from build123d import *

# Parameters (mm, degrees)
CLONE2D_W                = 34.6
CLONE2D_H                = 34.6
PAD004_DEPTH             = 1.2
SKETCH019_W              = 33
SKETCH019_H              = 33
PAD005_DEPTH             = 1.6
PAD006_DEPTH             = 3.3
SKETCH021_W              = 8
SKETCH021_H              = 22.4
SKETCH021_W_2            = 22.4
SKETCH021_H_2            = 5
SKETCH021_W_3            = 10
SKETCH021_H_3            = 9
POCKET014_DEPTH          = 1.2
SKETCH022_R              = 2.5
POCKET015_DEPTH          = 0.5
SKETCH023_R              = 1.25
POCKET016_DEPTH          = 6.101
SKETCH024_W              = 10.5
SKETCH024_H              = 4.5
SKETCH024_W_2            = 4.5
SKETCH024_H_2            = 8
SKETCH024_H_3            = 7
POCKET017_DEPTH          = 2.801
CLONE002_PLACEMENT_ANGLE = 180


with BuildPart() as part:
    # Clone2D → Pad004 (new body)
    with BuildSketch(Plane.XY):
        Rectangle(CLONE2D_W, CLONE2D_H)
    extrude(amount=PAD004_DEPTH)

    # Sketch019 → Pad005 (new body)
    with BuildSketch(Plane.XY.offset(1.2)):
        Rectangle(SKETCH019_W, SKETCH019_H)
    extrude(amount=PAD005_DEPTH)

    # Sketch020 → Pad006 (new body)
    with BuildSketch(Plane.XY.offset(2.8)):
        with BuildLine():
            ThreePointArc((-14, 11.5), (-12.232233, 12.232233), (-11.5, 14))
            Line((-11.5, 16.5), (-11.5, 14))
            Line((-11.5, 16.5), (-16.5, 16.5))
            Line((-16.5, 16.5), (-16.5, 11.5))
            Line((-16.5, 11.5), (-14, 11.5))
        make_face()
        with BuildLine():
            ThreePointArc((11.5, 14), (12.232233, 12.232233), (14, 11.5))
            Line((14, 11.5), (16.5, 11.5))
            Line((16.5, 11.5), (16.5, 16.5))
            Line((16.5, 16.5), (11.5, 16.5))
            Line((11.5, 16.5), (11.5, 14))
        make_face()
        with BuildLine():
            ThreePointArc((-11.5, -14), (-12.232233, -12.232233), (-14, -11.5))
            Line((-16.5, -11.5), (-14, -11.5))
            Line((-16.5, -16.5), (-16.5, -11.5))
            Line((-11.5, -16.5), (-16.5, -16.5))
            Line((-11.5, -14), (-11.5, -16.5))
        make_face()
        with BuildLine():
            ThreePointArc((14, -11.5), (12.232233, -12.232233), (11.5, -14))
            Line((11.5, -14), (11.5, -16.5))
            Line((11.5, -16.5), (16.5, -16.5))
            Line((16.5, -16.5), (16.5, -11.5))
            Line((16.5, -11.5), (14, -11.5))
        make_face()
    extrude(amount=PAD006_DEPTH)

    # Sketch021 → Pocket014 (cut)
    with BuildSketch(Plane.XY.offset(2.8)):
        with Locations((12.5, 0)):
            Rectangle(SKETCH021_W, SKETCH021_H)
        with Locations((0, -14)):
            Rectangle(SKETCH021_W_2, SKETCH021_H_2)
        with Locations((-9, 6.7)):
            Rectangle(SKETCH021_W_3, SKETCH021_H_3)
    extrude(amount=-POCKET014_DEPTH, mode=Mode.SUBTRACT)

    # Sketch022 → Pocket015 (cut)
    with BuildSketch(Plane(origin=(0, 0, 0), x_dir=(1, 0, 0), z_dir=(0, 0, -1))):
        with Locations((-14, 14)):
            Circle(SKETCH022_R)
        with Locations((14, 14)):
            Circle(SKETCH022_R)
        with Locations((-14, -14)):
            Circle(SKETCH022_R)
        with Locations((14, -14)):
            Circle(SKETCH022_R)
    extrude(amount=-POCKET015_DEPTH, mode=Mode.SUBTRACT)

    # Sketch023 → Pocket016 (cut, through all)
    with BuildSketch(Plane(origin=(0, 0, 0), x_dir=(1, 0, 0), z_dir=(0, 0, -1))):
        with Locations((-14, 14)):
            Circle(SKETCH023_R)
        with Locations((14, 14)):
            Circle(SKETCH023_R)
        with Locations((-14, -14)):
            Circle(SKETCH023_R)
        with Locations((14, -14)):
            Circle(SKETCH023_R)
    extrude(amount=-POCKET016_DEPTH, mode=Mode.SUBTRACT)

    # Sketch024 → Pocket017 (cut, through all)
    with BuildSketch(Plane.XY.offset(2.8)):
        with Locations((5.75, 15.25)):
            Rectangle(SKETCH024_W, SKETCH024_H)
        with Locations((-13.75, 4.7)):
            Rectangle(SKETCH024_W_2, SKETCH024_H_2)
        with Locations((13.75, -0.5)):
            Rectangle(SKETCH024_W_2, SKETCH024_H_3)
    extrude(amount=-POCKET017_DEPTH, mode=Mode.SUBTRACT)


with BuildPart() as part_1:
    # Clone002 placement: moved
    add(part.part.moved(Location((0, 0, 17.2))).rotate(Axis((0, 0, 17.2), (0, 1, 0)), CLONE002_PLACEMENT_ANGLE))


solid = part_1.part
Read the model definition and answer for the solid it produces. Units are mm, in the model's axes. A direction names the side the tool comes from. Coordinates: 2 decimals unless noted, no trailing zeros. Loops run counter-clockwise (first coordinate to the right, second up) from the corner with the lowest first, then second, coordinate; pieces in that order, holes last. Notation, with made-up numbers: (7.5, -35.5) -> (17.5, -35.5) arc R12 ccw to (17.5, -31.5) -> close; hole circle Ø3 at (6, 14). An arc over 180 degrees is marked (long way). Answer in a Markdown table with one row per item.
Item 1: For a pull along Y with two mould halves and no side action, classify faces 1 (the flat face through (11.5, -15, 13)), 2 (the cylindrical face through (12.252, 12.213, 12.773)), 3 (the flat face through (0, -17.3, 17)) as released by +Y, released by -Y, zero draft, split by the parting line, or undercut.
Returned:
| item | result |
|---|---|
| face 1 | zero draft |
| face 2 | undercut |
| face 3 | released by -Y |
Item 2: Straight lines are drawn through the part: line 1 along Y through (x, z) = (-14, 14.85); line 2 along Y through (x, z) = (-14, 13.6). For each, find the intervals that lie inside material, in ascending order. Write a range as [from, to].
Returned:
| item | result |
|---|---|
| line 1 | y = [-16.5, -15.25], [-12.75, -11.2], [11.2, 12.75], [15.25, 16.5] |
| line 2 | y = [-16.5, -15.25], [-12.75, -11.5], [11.5, 12.75], [15.25, 16.5] |
Item 3: A cutting plane is placed at C-C on x = -10. Determine the outline of the cut face in (y, z), plus the area to 3 significant figures.
Returned:
| item | result |
|---|---|
| outline | (-17.3, 16) -> (-16.5, 16) -> (-16.5, 15.6) -> (-11.5, 15.6) -> (-11.5, 14.4) -> (-11.2, 14.4) -> (-11.2, 15.6) -> (11.2, 15.6) -> (11.2, 14.4) -> (13, 14.4) -> (13, 17.2) -> (-17.3, 17.2) -> close |
| area | 50.7 mm^2 |
Item 4: A cutting plane is placed at B-B on y = 4.5. Determine the outline of the cut face in (x, z), plus the area to 3 significant figures.
Returned:
| item | result |
|---|---|
| outline | (-17.3, 16) -> (-16.5, 16) -> (-16.5, 15.6) -> (-8.5, 15.6) -> (-8.5, 14.4) -> (4, 14.4) -> (4, 15.6) -> (11.5, 15.6) -> (11.5, 17.2) -> (-17.3, 17.2) -> close; (16, 14.4) -> (16.5, 14.4) -> (16.5, 16) -> (17.3, 16) -> (17.3, 17.2) -> (16, 17.2) -> close |
| area | 63.1 mm^2 |
Item 5: Each of these flat-tipped pins is pushed along its axis until it touches: P1, Ø1.5, axis at x = 3.5, y = 3.5, coming from the -Z side; P2, Ø2.5, axis at y = 1.5, z = 14.5, coming from the +X side; P3, Ø2.5, axis at x = 10.5, z = 14.5, coming from the +Y side; P4, Ø1.5, axis at x = 2.5, z = 12, coming from the -Y side. Where does it stop, or does it pass through?
Returned:
| item | result |
|---|---|
| P1 | stops at z = 14.4 |
| P2 | stops at x = 16.5 |
| P3 | stops at y = 16.5 |
| P4 | passes through |
Item 6: For faces 4 (the flat face through (0, -11.5, 15)), 5 (the flat face through (-14, -4, 16)), 6 (the flat face through (15, -13, 16.7)), 7 (the flat face through (-15, -11.5, 13)), 8 (the flat face through (16.5, 0, 15)), determine the directions among +Z, -Z, +X, -X, +Y, -Y from which every point of the face is accessible in a straight line to the end or side of a thin tool.
Returned:
| item | result |
|---|---|
| face 4 | -Z, -Y |
| face 5 | +Z, -Z |
| face 6 | +Z |
| face 7 | -Z, +X, -X |
| face 8 | -Z, +X, +Y, -Y |
Item 7: A cutting plane is placed at A-A on z = 13.25. Determine the outline of the cut face in (x, y), plus the area to 3 significant figures.
Returned:
| item | result |
|---|---|
| outline | (-16.5, -16.5) -> (-11.5, -16.5) -> (-11.5, -14) arc R2.5 ccw to (-14, -11.5) -> (-16.5, -11.5) -> close; (-16.5, 11.5) -> (-14, 11.5) arc R2.5 ccw to (-11.5, 14) -> (-11.5, 16.5) -> (-16.5, 16.5) -> close; (11.5, -16.5) -> (16.5, -16.5) -> (16.5, -11.5) -> (14, -11.5) arc R2.5 ccw to (11.5, -14) -> close; (11.5, 14) arc R2.5 ccw to (14, 11.5) -> (16.5, 11.5) -> (16.5, 16.5) -> (11.5, 16.5) -> close; hole circle Ø2.5 at (-14, -14); hole circle Ø2.5 at (-14, 14); hole circle Ø2.5 at (14, -14); hole circle Ø2.5 at (14, 14) |
| area | 75.0 mm^2 |
Item 8: A cutting plane is placed at D-D on x = 9.5. Determine the outline of the cut face in (y, z), plus the area to 3 significant figures.
Returned:
| item | result |
|---|---|
| outline | (-17.3, 16) -> (-16.5, 16) -> (-16.5, 15.6) -> (-11.5, 15.6) -> (-11.5, 14.4) -> (2.2, 14.4) -> (2.2, 15.6) -> (11.2, 15.6) -> (11.2, 14.4) -> (16.5, 14.4) -> (16.5, 16) -> (17.3, 16) -> (17.3, 17.2) -> (-17.3, 17.2) -> close |
| area | 77.5 mm^2 |
